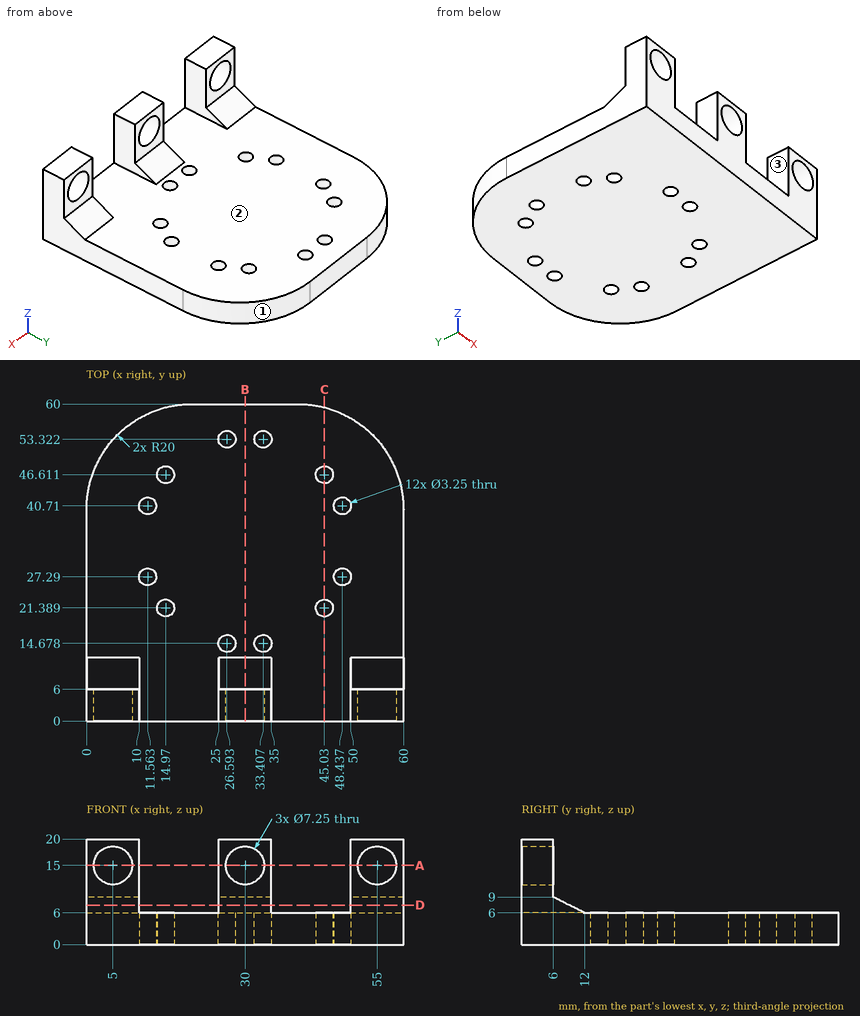
Study the drawing (mm; zero at the part's minimum x, y, z) and answer. A direction names the side the tool comes from. Round coordinates to 2 decimals unless told otherwise and drop trailing zeros. Loops run counter-clockwise (first coordinate to the right, second up) from the corner with the lowest first, then second, coordinate; pieces in that order, holes last.
Q1. Which of the six approach directions +Z, -Z, +X, -X, +Y, -Y give full straight-line access (tool end or side, diameter ignored) to the marked faces 1, 2 and 3?
Q2. Section A-A, the plane z = 15 is taken. Determine the outline of the cut face in (x, y) (1 decimal).
Q3. Section C-C, the plane x = 45 is taken. Determine the outline of the cut face in (y, z) (1 decimal), then the cut area to 3 significant figures.
Q4. Section D-D, the plane z = 7.5 is taken. Determine the outline of the cut face in (x, y), then the cut area to 3 significant figures.
Q5. Find the intervals of material crossed by line 1 (X direction, y = 2.5, z = 15) (1 decimal); line 2 (Z direction, x = 5, y = 2.25) (1 decimal); line 3 (Y direction, x = 26, z = 13.5), in increasing order.
Q6. Section B-B, the plane x = 30 is taken. Determine the outline of the cut face in (y, z) (1 decimal).
Q7. Given pin 1 Ø3.5 at (x, y) = (14.97, 46.61) entering from +Z; pin 2 Ø6 at (x, y) = (40.5, 35) entering from -Z; pin 3 Ø3 at (x, z) = (57, 15) entering from +Y; pin 4 Ø8.5 at (x, z) = (30, 15) entering from +Y, each flat-ended and moving along its own axis, determine where each tip first touches the part or whether it passes through.
Completed:
1. face 1: +Z, -Z, +X, +Y
1. face 2: +Z, +Y
1. face 3: +Z, +Y, -Y
2. outline: (0, 0) - (1.4, 0) - (1.4, 6) - (0, 6) - close; (8.6, 0) - (10, 0) - (10, 6) - (8.6, 6) - close; (25, 0) - (26.4, 0) - (26.4, 6) - (25, 6) - close; (33.6, 0) - (35, 0) - (35, 6) - (33.6, 6) - close; (50, 0) - (51.4, 0) - (51.4, 6) - (50, 6) - close; (58.6, 0) - (60, 0) - (60, 6) - (58.6, 6) - close
3. outline: (0, 0) - (19.8, 0) - (19.8, 6) - (0, 6) - close; (23, 0) - (45, 0) - (45, 6) - (23, 6) - close; (48.2, 0) - (59.4, 0) - (59.4, 6) - (48.2, 6) - close
3. area: 317 mm2
4. outline: (0, 0) - (10, 0) - (10, 9) - (0, 9) - close; (25, 0) - (35, 0) - (35, 9) - (25, 9) - close; (50, 0) - (60, 0) - (60, 9) - (50, 9) - close
4. area: 270 mm2
5. line 1: x = 0 to 1.4, 8.6 to 10, 25 to 26.4, 33.6 to 35, 50 to 51.4, 58.6 to 60
5. line 2: z = 0 to 11.4, 18.6 to 20
5. line 3: y = 0 to 6
6. outline: (0, 0) - (60, 0) - (60, 6) - (12, 6) - (6, 9) - (6, 11.4) - (0, 11.4) - close; (0, 18.6) - (6, 18.6) - (6, 20) - (0, 20) - close
7. pin 1: stops at z = 6
7. pin 2: stops at z = 0
7. pin 3: passes through
7. pin 4: stops at y = 6
